from build123d import *

# Parameters (mm, degrees)
SKETCH1_R           = 19.05
SKETCH1_R_2         = 13.97
BOSS_EXTRUDE1_DEPTH = 7.62
SKETCH2_R           = 1.5875
CUT_EXTRUDE1_DEPTH  = 28.99766776
CUT_EXTRUDE2_START  = -5.08
SKETCH3_R           = 1.5875
CUT_EXTRUDE2_DEPTH  = 5.08
SKETCH4_R           = 1.5
CUT_EXTRUDE3_DEPTH  = 28.99766776
SKETCH5_R           = 2
CUT_EXTRUDE4_DEPTH  = 5.7
SKETCH6_R           = 4
SKETCH6_R_2         = 2
BOSS_EXTRUDE2_DEPTH = 7.62
CIRPATTERN1_COUNT   = 4


with BuildPart() as part:
    # Sketch1 → Boss-Extrude1 (new body)
    with BuildSketch(Plane.XY):
        with Locations(Location((0, 0, 0), (0, 0, 180))):
            Circle(SKETCH1_R)
        with Locations(Location((0, 0, 0), (0, 0, 180))):
            Circle(SKETCH1_R_2, mode=Mode.SUBTRACT)
    extrude(amount=BOSS_EXTRUDE1_DEPTH)

    # Sketch2 → Cut-Extrude1 (cut, through all)
    with BuildSketch(Plane.XY.offset(7.62)):
        with Locations((0, 16.51)):
            Circle(SKETCH2_R)
        with Locations((16.51, 0)):
            Circle(SKETCH2_R)
        with Locations((0, -16.51)):
            Circle(SKETCH2_R)
        with Locations((-16.51, 0)):
            Circle(SKETCH2_R)
    extrude(amount=-CUT_EXTRUDE1_DEPTH, mode=Mode.SUBTRACT)

    # Sketch3 → Cut-Extrude2 (cut)
    # profile 1 of 4: a face of its own
    with BuildSketch(Plane.XY.offset(7.62).offset(CUT_EXTRUDE2_START)):
        with BuildLine():
            ThreePointArc((-18.783553311, 3.175), (-19.05, 0), (-18.783553311, -3.175))
            Line((-18.783553311, -3.175), (-13.604421156, -3.175))
            ThreePointArc((-13.604421156, -3.175), (-13.97, 0), (-13.604421156, 3.175))
            Line((-13.604421156, 3.175), (-18.783553311, 3.175))
        make_face()
        with Locations((-16.51, 0)):
            Circle(SKETCH3_R, mode=Mode.SUBTRACT)
    # profile 2 of 4: a face of its own
    with BuildSketch(Plane.XY.offset(7.62).offset(CUT_EXTRUDE2_START)):
        with BuildLine():
            Line((-3.175, -13.604421156), (-3.175, -18.783553311))
            ThreePointArc((-3.175, -18.783553311), (0, -19.05), (3.175, -18.783553311))
            Line((3.175, -18.783553311), (3.175, -13.604421156))
            ThreePointArc((3.175, -13.604421156), (0, -13.97), (-3.175, -13.604421156))
        make_face()
        with Locations((0, -16.51)):
            Circle(SKETCH3_R, mode=Mode.SUBTRACT)
    # profile 3 of 4: a face of its own
    with BuildSketch(Plane.XY.offset(7.62).offset(CUT_EXTRUDE2_START)):
        with BuildLine():
            Line((13.604421156, -3.175), (18.783553311, -3.175))
            ThreePointArc((18.783553311, -3.175), (18.983271459, -1.593080258), (19.05, 0))
            ThreePointArc((19.05, 0), (18.983271459, 1.593080258), (18.783553311, 3.175))
            Line((18.783553311, 3.175), (13.604421156, 3.175))
            ThreePointArc((13.604421156, 3.175), (13.878304355, 1.597988806), (13.97, 0))
            ThreePointArc((13.97, 0), (13.878304355, -1.597988806), (13.604421156, -3.175))
        make_face()
        with Locations((16.51, 0)):
            Circle(SKETCH3_R, mode=Mode.SUBTRACT)
    # profile 4 of 4: a face of its own
    with BuildSketch(Plane.XY.offset(7.62).offset(CUT_EXTRUDE2_START)):
        with BuildLine():
            ThreePointArc((3.175, 18.783553311), (0, 19.05), (-3.175, 18.783553311))
            Line((-3.175, 18.783553311), (-3.175, 13.604421156))
            ThreePointArc((-3.175, 13.604421156), (0, 13.97), (3.175, 13.604421156))
            Line((3.175, 13.604421156), (3.175, 18.783553311))
        make_face()
        with Locations((0, 16.51)):
            Circle(SKETCH3_R, mode=Mode.SUBTRACT)
    extrude(amount=CUT_EXTRUDE2_DEPTH, mode=Mode.SUBTRACT)

    # Sketch4 → Cut-Extrude3 (cut, through all)
    with BuildSketch(Plane.XY.offset(7.62)):
        with Locations((-11.674332957, 11.674332957)):
            Circle(SKETCH4_R)
    cut_extrude3 = extrude(amount=-CUT_EXTRUDE3_DEPTH, mode=Mode.SUBTRACT)

    # Sketch5 → Cut-Extrude4 (cut)
    with BuildSketch(Plane.XY.offset(7.62)):
        with Locations((-11.674332957, 11.674332957)):
            Circle(SKETCH5_R)
    cut_extrude4 = extrude(amount=-CUT_EXTRUDE4_DEPTH, mode=Mode.SUBTRACT)

    # Sketch6 → Boss-Extrude2 (add)
    with BuildSketch(Plane.XY.offset(7.62)):
        with Locations((-11.674332957, 11.674332957)):
            Circle(SKETCH6_R)
        with Locations((-11.674332957, 11.674332957)):
            Circle(SKETCH6_R_2, mode=Mode.SUBTRACT)
    boss_extrude2 = extrude(amount=-BOSS_EXTRUDE2_DEPTH)

    # CirPattern1: Cut-Extrude3, Cut-Extrude4, Boss-Extrude2 ×4 about axis
    cirpattern1_axis = Axis((0, 0, 0), (0, 0, 1))
    add([cut_extrude3.rotate(cirpattern1_axis, i * 360 / CIRPATTERN1_COUNT) for i in range(1, CIRPATTERN1_COUNT)], mode=Mode.SUBTRACT)
    add([cut_extrude4.rotate(cirpattern1_axis, i * 360 / CIRPATTERN1_COUNT) for i in range(1, CIRPATTERN1_COUNT)], mode=Mode.SUBTRACT)
    add([boss_extrude2.rotate(cirpattern1_axis, i * 360 / CIRPATTERN1_COUNT) for i in range(1, CIRPATTERN1_COUNT)])


solid = part.part
Verification items for the finished model (mm, model axes). A direction names the side the tool comes from. Give positions to 0.01 mm unless a question says otherwise; leave off trailing zeros. Order: outer loops, then holes, each group sorted by start corner. A loop starts at its lowest first (then second) coordinate and runs counter-clockwise, first axis right, second up. Notation, with made-up numbers: M 32,12.5 L 47,12.5 A18 ccw 47,28.5 Z; hole C 35,41 d9. An arc over 180 degrees is marked long. Use one line per item in the form item = value. Start each with the question number.
Q1. Scan lines: line 1 along Y through (x, z) = (0, 1.7); line 2 along X through (y, z) = (-10, 5); line 3 along X through (y, z) = (11, 6.75). Record each from-to range of solid material in increasing order. Write a range as [from, to].
Q2. Go/stop test with flat-tipped pins: pin 1 Ø4 at (x, z) = (-15.5, 5.5) entering from -Y; pin 2 Ø1.6 at (x, y) = (0.5, 17.5) entering from +Z; pin 3 Ø3 at (x, y) = (12, -12) entering from +Z; pin 4 Ø1.2 at (x, y) = (11.5, 11.5) entering from +Z. Record where each tip stops, or that it passes through.
Q3. Section check A-A (x = 0). Enter the section's corners in (y, z).
Q4. Access from +Z, -Z, +X, -X, +Y, -Y to the whole of each face (thin tool, end or side, straight path). Record for faces 1 (the cylindrical face through (19.05, -0.16, 2.06)), 2 (the cylindrical face through (-9.827, 10.908, 4.81)), 3 (the cylindrical face through (-8.88, 8.81, 3.86)), 4 (the flat face through (-16, -3.175, 5)).
Q5. Section check C-C (y = -6). Enter the section's corners in (x, z), then the cut area to 3 significant figures.
Q6. Section check D-D (x = -6.5). Enter the section's corners in (y, z).
Q7. Mould release check, pull along Y, two halves, no side actions. Record for faces 5 (the flat face through (9, -10, 0)), 6 (the cylindrical face through (13.97, -0.11, 2.06)): +Y half, -Y half, draft (parallel to the pull), parting line (faces both ways), or undercut.
Evaluation:
q1.line_1 = [-19.05, -18.1], [-14.92, -13.97], [13.97, 14.92], [18.1, 19.05]
q1.line_2 = [-16.21, -12.77], [-10.58, -8.04], [8.04, 10.58], [12.77, 16.21]
q1.line_3 = [-15.62, -13.56], [-9.79, -7.73], [7.73, 9.79], [13.56, 15.62]
q2.pin_1 = -15.23
q2.pin_2 = 2.54
q2.pin_3 = 1.92
q2.pin_4 = through
q3.outline = M -19.05,0 L -18.1,0 L -18.1,2.54 L -19.05,2.54 Z; M -14.92,0 L -13.97,0 L -13.97,2.54 L -14.92,2.54 Z; M 13.97,0 L 14.92,0 L 14.92,2.54 L 13.97,2.54 Z; M 18.1,0 L 19.05,0 L 19.05,2.54 L 18.1,2.54 Z
q4.face_1 = +Z, -Z, +X
q4.face_2 = +Z
q4.face_3 = +Z, -Z
q4.face_4 = +Z, +X, -X
q5.outline = M -18.08,0 L -12.62,0 L -12.62,7.62 L -18.08,7.62 Z; M 12.62,0 L 18.08,0 L 18.08,7.62 L 12.62,7.62 Z
q5.area = 83.3 mm2
q6.outline = M -17.91,0 L -12.37,0 L -12.37,7.62 L -17.91,7.62 Z; M 12.37,0 L 17.91,0 L 17.91,7.62 L 12.37,7.62 Z
q7.face_5 = draft
q7.face_6 = undercut
